Verification items for the finished model (mm, model axes). A direction names the side the tool comes from. Give positions to 0.01 mm unless a question says otherwise; leave off trailing zeros. Loops run counter-clockwise (first coordinate to the right, second up) from the corner with the lowest first, then second, coordinate; pieces in that order, holes last. Notation, with made-up numbers: (-19, -3.5) - (19, -3.5) arc R23 cw to (19, 6.5) - close; hole circle Ø2 at (40, 69.25). An arc over 180 degrees is marked (long way). One line per item, written item: value. Start each with the question number.
1. Sectioned sample at C-C (y = 9). Record the cut outline in (x, z).
2. Gauge pin test, flat ends, axial feed: pin 1 (8 mm diameter, centred on y = 20, z = 4.5, fed in from +X); pin 2 (3 mm diameter, centred on x = 16, z = -2.5, fed in from -Y); pin 3 (4 mm diameter, centred on y = 12, z = 1.5, fed in from -X); pin 4 (4 mm diameter, centred on y = 6.5, z = -5.5, fed in from -X). Record the tip position at first contact, or that the pin passes through.
3. Sectioned sample at B-B (x = -40). Record the cut outline in (y, z).
4. Access from +Z, -Z, +X, -X, +Y, -Y to the whole of each face (thin tool, end or side, straight path). Record for faces 1 (the flat face through (-2, 2, 5)), 2 (the flat face through (-120, 2, 0)), 3 (the flat face through (-118, 2, 0)), 4 (the flat face through (118.3, 5, -0.1)), 5 (the flat face through (-118.4, 5, -0.1)).
5. Sectioned sample at A-A (z = 1). Record the cut outline in (x, y).
6. Scan lines: L1, parallel to Z at x = 104, y = 2.5; L2, parallel to X at y = 2, z = -2.5; L3, parallel to X at y = 5.5, z = 3.75. Record each from-to range of solid material in increasing order. Write a range as [from, to].
from build123d import *

# Parameters (mm, degrees)
SKETCH1_W           = 240
SKETCH1_H           = 16
BOSS_EXTRUDE1_DEPTH = 5
SKETCH2_W           = 236
SKETCH2_H           = 10
CUT_EXTRUDE1_DEPTH  = 5
SKETCH4_W           = 220
SKETCH4_H           = 16
BOSS_EXTRUDE3_DEPTH = 20


with BuildPart() as part:
    # Sketch1 → Boss-Extrude1 (new body)
    with BuildSketch(Plane(origin=(0, 0, 0), x_dir=(1, 0, 0), z_dir=(0, 1, 0))):
        Rectangle(SKETCH1_W, SKETCH1_H)
    extrude(amount=BOSS_EXTRUDE1_DEPTH)

    # Sketch2 → Cut-Extrude1 (cut)
    with BuildSketch(Plane(origin=(0, 0, 0), x_dir=(1, 0, 0), z_dir=(0, 1, 0))):
        Rectangle(SKETCH2_W, SKETCH2_H)
    extrude(amount=CUT_EXTRUDE1_DEPTH, mode=Mode.SUBTRACT)

    # Sketch4 → Boss-Extrude3 (add)
    with BuildSketch(Plane(origin=(0, 5, 0), x_dir=(1, 0, 0), z_dir=(0, 1, 0))):
        Rectangle(SKETCH4_W, SKETCH4_H)
    extrude(amount=BOSS_EXTRUDE3_DEPTH)


solid = part.part
Results are:
1. outline: (-110, -8) - (110, -8) - (110, 8) - (-110, 8) - close
2. pin 1: stops at x = 110
2. pin 2: stops at y = 5
2. pin 3: stops at x = -110
2. pin 4: stops at x = -120
3. outline: (0, -8) - (25, -8) - (25, 8) - (0, 8) - (0, 5) - (5, 5) - (5, -5) - (0, -5) - close
4. face 1: -Y
4. face 2: +Z, -Z, -X, +Y, -Y
4. face 3: +Y, -Y
4. face 4: +Z, -Z, +X, +Y
4. face 5: +Z, -Z, -X, +Y
5. outline: (-120, 0) - (-118, 0) - (-118, 5) - (-120, 5) - close; (-110, 5) - (110, 5) - (110, 25) - (-110, 25) - close; (118, 0) - (120, 0) - (120, 5) - (118, 5) - close
6. L1: z = [-8, -5], [5, 8]
6. L2: x = [-120, -118], [118, 120]
6. L3: x = [-110, 110]
